Read the model definition and answer for the solid it produces. Units are mm, in the model's axes. A direction names the side the tool comes from. Coordinates: 2 decimals unless noted, no trailing zeros. Loops run counter-clockwise (first coordinate to the right, second up) from the corner with the lowest first, then second, coordinate; pieces in that order, holes last. Notation, with made-up numbers: M -1,-40 L 42,-40 A6 ccw 42,-29 Z; hole C 1,40.25 d8. An arc over 180 degrees is marked long. Put each result on its own line as item: value.
from build123d import *

# Parameters (mm, degrees)
PAD_DEPTH = 2


with BuildPart() as part:
    # Sketch → Pad (new body)
    with BuildSketch(Plane.XY):
        with BuildLine():
            ThreePointArc((-27.489858, -0.746794), (27.360019, -2.771163), (-26.781824, 6.243707))
            ThreePointArc((-26.781824, 6.243707), (-26.728683, 3.219003), (-25.249794, 0.579962))
            Line((-25.249794, 0.579962), (-15.435404, -9.800129))
            ThreePointArc((-15.435404, -9.800129), (-14.079498, -9.894335), (-13.873578, -8.55085))
            Line((-13.873578, -8.55085), (-19.209537, -0.614914))
            ThreePointArc((-19.887258, 2.120607), (-19.789586, 0.693092), (-19.209537, -0.614914))
            ThreePointArc((-18.249364, -8.182952), (19.751995, 3.139854), (-19.887258, 2.120607))
            ThreePointArc((-18.249364, -8.182952), (-19.207091, -6.452486), (-20.440588, -4.906446))
            Line((-20.440588, -4.906446), (-25.249794, 0.179962))
            ThreePointArc((-25.249794, 0.179962), (-26.688775, 0.487518), (-27.489858, -0.746794))
        make_face()
    extrude(amount=PAD_DEPTH)


solid = part.part
1) Which of the six approach directions +Z, -Z, +X, -X, +Y, -Y give full straight-line access (tool end or side, diameter ignored) to faces 4 (the cylindrical face through (-19.19, -6.48, 0.99)), 5 (the flat face through (-18.7, -5.7, 2))?
Answer list:
face 4: +Z, -Z
face 5: +Z, +X, -X, +Y, -Y
2) Find section D-D, the plane y = 23. Write down the section's boundary in (x, z).
Answer list:
outline: M -15.07,0 L 15.07,0 L 15.07,2 L -15.07,2 Z
3) Find section B-B, the plane y = 8. Write down the section's boundary in (x, z).
Answer list:
outline: M -26.31,0 L -18.33,0 L -18.33,2 L -26.31,2 Z; M 18.33,0 L 26.31,0 L 26.31,2 L 18.33,2 Z
4) Find section C-C, the plane z = 0.6. Write down the section's boundary in (x, y), plus the area to 3 significant figures.
Answer list:
outline: M -27.49,-0.75 A27.5 ccw long -26.78,6.24 A6.2 ccw -25.25,0.58 L -15.44,-9.8 A1 ccw -13.87,-8.55 L -19.21,-0.61 A4.12 cw -19.89,2.12 A20 cw long -18.25,-8.18 A11.79 ccw -20.44,-4.91 L -25.25,0.18 A1.3 ccw Z
area: 1,140 mm^2
5) Straight lines are drawn through the part: line 1 (Y direction, x = 0, z = 0.7); line 2 (X direction, y = -3.5, z = 0.65); line 3 (X direction, y = 0, z = 0.7). For each, find the intervals that lie inside material, in ascending order. Write a range as [from, to].
Answer list:
line 1: y = [-27.5, -20], [20, 27.5]
line 2: x = [-27.28, -21.77], [-21.39, -17.27], [19.69, 27.28]
line 3: x = [-27.28, -25.08], [-24.7, -19.55], [20, 27.5]
6) Determine the mould class of faces 1 (the cylindrical face through (27.22, -3.92, 0.99)), 2 (the flat face through (-20.41, -4.54, 0.99)), 3 (the flat face through (-18.7, -5.7, 0)) for opening direction Y: released by +Y, released by -Y, zero draft, split by the parting line, or undercut.
Answer list:
face 1: split by the parting line
face 2: undercut
face 3: zero draft
7) Given pin 1 Ø1 at (x, z) = (5, 1) entering from -Y; pin 2 Ø1 at (y, z) = (-15, 1) entering from +X, each flat-ended and moving along its own axis, determine where each tip first touches the part or whether it passes through.
Answer list:
pin 1: stops at y = -27.13
pin 2: stops at x = 23.37
8) Find section A-A, the plane x = 0. Write down the section's boundary in (y, z).
Answer list:
outline: M -27.5,0 L -20,0 L -20,2 L -27.5,2 Z; M 20,0 L 27.5,0 L 27.5,2 L 20,2 Z
